from build123d import *

# Parameters (mm, degrees)
BOSS_EXTRUDE1_DEPTH         = 25.4
M3X0_5_TAPPED_HOLE1_D       = 2.5
F_1_4_20_TAPPED_HOLE1_D     = 5.1054
F_1_4_20_TAPPED_HOLE1_DEPTH = 6.35
FILLET1_R                   = 2.54
FILLET2_R                   = 0.254


with BuildPart() as part:
    # Sketch1 → Boss-Extrude1 (new body)
    with BuildSketch(Plane.XY):
        Polygon((69.85, 69.85), (69.85, 76.2), (0, 76.2), (0, 0), (69.85, 0), (69.85, 6.35), (6.35, 6.35), (6.35, 69.85), align=None)
    extrude(amount=BOSS_EXTRUDE1_DEPTH)

    # M3x0.5 Tapped Hole1 (through all)
    with Locations(Plane.ZY):
        with Locations((12.7, 57.15), (12.7, 38.1), (12.7, 19.05)):
            Hole(M3X0_5_TAPPED_HOLE1_D / 2)

    # 1/4-20 Tapped Hole1
    with Locations(Plane(origin=(0, 0, 0), x_dir=(-1, 0, 0), z_dir=(0, -1, 0))):
        with Locations((-38.1, -12.7)):
            Hole(F_1_4_20_TAPPED_HOLE1_D / 2, depth=F_1_4_20_TAPPED_HOLE1_DEPTH)

    # Fillet1
    fillet1_edges = [part.edges().sort_by_distance(p)[0] for p in [
        (69.85, 3.175, 0),
        (69.85, 3.175, 25.4),
        (69.85, 73.025, 25.4),
        (69.85, 73.025, 0),
    ]]
    fillet(fillet1_edges, radius=FILLET1_R)

    # Fillet2
    fillet2_edges = [part.edges().sort_by_distance(p)[0] for p in [
        (33.655, 0, 0),
        (6.35, 38.1, 25.4),
        (69.85, 6.35, 12.7),
        (69.85, 0, 12.7),
        (36.83, 6.35, 0),
        (36.83, 6.35, 25.4),
        (69.106051224, 6.35, 24.656051224),
        (69.106051224, 6.35, 0.743948776),
        (33.655, 76.2, 0),
        (69.106051224, 0, 24.656051224),
        (69.106051224, 0, 0.743948776),
        (33.655, 76.2, 25.4),
        (69.85, 76.2, 12.7),
        (69.106051224, 76.2, 24.656051224),
        (69.106051224, 76.2, 0.743948776),
        (33.655, 0, 25.4),
        (6.35, 38.1, 0),
    ]]
    fillet(fillet2_edges, radius=FILLET2_R)


solid = part.part
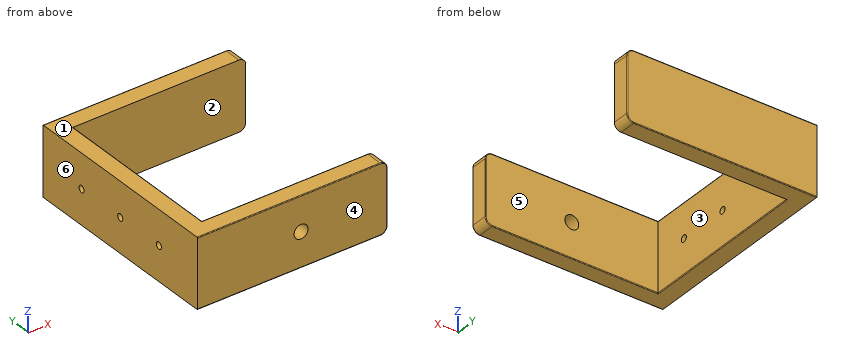
The model under review builds one solid part; all positions refer to its coordinate system, in mm. Face numbers are marked on the shaded views. A direction names the side the tool comes from. Round coordinates to 2 decimals unless told otherwise and drop trailing zeros. Write each loop counter-clockwise with the first axis right and the second up, starting at its lowest first coordinate (ties: lowest second). Pieces come first, ordered by that corner, then holes. Notation, with made-up numbers: M 1,-3 L 37,-3 A19 cw 37,33 Z; hole C 52.25,-3 d7. An arc over 180 degrees is marked long. Answer as CSV lines item,"result". Start each with the question number.
Q1. Consider section B-B, the plane x = 38.1. Give the boundary of the cut face in (y, z).
Q2. Wall thickness on line 1 along Y through (x, z) = (1.75, 12.7); line 2 along Y through (x, z) = (32, 10.25); line 3 along Z through (x, y) = (38.1, 4): over which ranges is each line inside the solid? List them lowest first.
Q3. The part is to be moulded in two halves that separate along Y. For the marked faces 3, 4, 5 and 6, say which applies: +Y half, -Y half, draft (parallel to the pull), parting line (faces both ways), or undercut.
Q4. Consider section A-A, the plane z = 12.7. Give the boundary of the cut face in (x, y).
Q5. Consider section D-D, the plane x = 9. Give the boundary of the cut face in (y, z), then the cut area to 3 significant figures.
Q6. Clearance check with flat-ended pins moving along their axes: P1, Ø2, axis at y = 38.1, z = 12.7, coming from the +X side; P2, Ø8, axis at y = 55.5, z = 5, coming from the +X side. State where each tip first meets the part, or that it passes through.
Q7. Tool access review of the marked faces 1 and 2: name each direction out of +Z, -Z, +X, -X, +Y, -Y from which nothing blocks a thin tool from reaching the whole face with its end or side.
Q8. Consider section C-C, the plane y = 57.15. Give the boundary of the cut face in (x, z), then the cut area to 3 significant figures.
Result set:
1,outline,"M 0,0.25 A0.25 ccw 0.25,0 L 6.1,0 A0.25 ccw 6.35,0.25 L 6.35,10.15 L 0,10.15 Z; M 0,15.25 L 6.35,15.25 L 6.35,25.15 A0.25 ccw 6.1,25.4 L 0.25,25.4 A0.25 ccw 0,25.15 Z; M 69.85,0 L 75.95,0 A0.25 ccw 76.2,0.25 L 76.2,25.15 A0.25 ccw 75.95,25.4 L 69.85,25.4 Z"
2,line 1,"y = 0 to 17.8, 20.3 to 36.85, 39.35 to 55.9, 58.4 to 76.2"
2,line 2,"y = 0 to 6.35, 69.85 to 76.2"
2,line 3,"z = 0 to 10.15, 15.25 to 25.4"
3,face 3,"undercut"
3,face 4,"-Y half"
3,face 5,"undercut"
3,face 6,"draft"
4,outline,"M 0,0 L 35.55,0 L 35.55,6.35 L 6.35,6.35 L 6.35,17.8 L 0,17.8 Z; M 0,20.3 L 6.35,20.3 L 6.35,36.85 L 0,36.85 Z; M 0,39.35 L 6.35,39.35 L 6.35,55.9 L 0,55.9 Z; M 0,58.4 L 6.35,58.4 L 6.35,69.85 L 69.85,69.85 L 69.85,75.95 A0.25 ccw 69.6,76.2 L 0,76.2 Z; M 40.65,0 L 69.6,0 A0.25 ccw 69.85,0.25 L 69.85,6.1 A0.25 ccw 69.6,6.35 L 40.65,6.35 Z"
5,outline,"M 0,0.25 A0.25 ccw 0.25,0 L 6.1,0 A0.25 ccw 6.35,0.25 L 6.35,25.15 A0.25 ccw 6.1,25.4 L 0.25,25.4 A0.25 ccw 0,25.15 Z; M 69.85,0 L 75.95,0 A0.25 ccw 76.2,0.25 L 76.2,25.15 A0.25 ccw 75.95,25.4 L 69.85,25.4 Z"
5,area,"322 mm²"
6,P1,"passes through"
6,P2,"stops at x = 6.35"
7,face 1,"+Z, +X, -X, +Y, -Y"
7,face 2,"+Z, -Z, +X"
8,outline,"M 0,0 L 6.1,0 A0.25 ccw 6.35,0.25 L 6.35,11.45 L 0,11.45 Z; M 0,13.95 L 6.35,13.95 L 6.35,25.15 A0.25 ccw 6.1,25.4 L 0,25.4 Z"
8,area,"145 mm²"
